The listing builds one solid part. Answer for the finished solid, in the listing's coordinates (mm). A direction names the side the tool comes from. Coordinates: 2 decimals unless noted, no trailing zeros. Write each loop counter-clockwise with the first axis right and the second up, starting at its lowest first coordinate (ties: lowest second). Pieces come first, ordered by that corner, then holes.
(1) Which of the six approach directions +Z, -Z, +X, -X, +Y, -Y give full straight-line access (tool end or side, diameter ignored) to faces 1 (the flat face through (36.512, 6, 129)), 2 (the flat face through (38.1, 6, 125))?
(2) The part is cut by section D-D on z = 50.5. Determine the outline of the cut face in (x, y), plus the area to 3 significant figures.
(3) The part is cut by section B-B on x = 20. Determine the outline of the cut face in (y, z).
(4) The part is cut by section A-A on x = 7. Determine the outline of the cut face in (y, z), plus the area to 3 significant figures.
(5) Straight lines are drawn through the part: line 1 (X direction, y = 8.25, z = 152); line 2 (Y direction, x = 16.5, z = 80.5). For each, find the intervals that lie inside material, in ascending order.
(6) The part is cut by section C-C on y = 5.5. Determine the outline of the cut face in (x, z).
(7) For a pull along X with two mould halves and no side action, classify faces 3 (the flat face through (0, 6, 125)), 4 (the flat face through (18, 1, 0)), 5 (the flat face through (19, 11.112, 129)) as +X half, -X half, draft (parallel to the pull), parting line (faces both ways), or undercut.
from build123d import *

# Parameters (mm, degrees)
SKETCH1_W           = 38.1
SKETCH1_H           = 12.7
BOSS_EXTRUDE1_DEPTH = 254
SKETCH2_W           = 34.925
SKETCH2_H           = 9.525
CUT_EXTRUDE1_DEPTH  = 258.155400488
CUT_EXTRUDE2_DEPTH  = 258.155400488


with BuildPart() as part:
    # Sketch1 → Boss-Extrude1 (new body)
    with BuildSketch(Plane.XY):
        with Locations((19.05, 6.35)):
            Rectangle(SKETCH1_W, SKETCH1_H)
    extrude(amount=BOSS_EXTRUDE1_DEPTH)

    # Sketch2 → Cut-Extrude1 (cut, through all)
    with BuildSketch(Plane.XY.offset(254)):
        with Locations((19.05, 6.35)):
            Rectangle(SKETCH2_W, SKETCH2_H)
    extrude(amount=-CUT_EXTRUDE1_DEPTH, mode=Mode.SUBTRACT)

    # Sketch3 → Cut-Extrude2 (cut, through all)
    with BuildSketch(Plane.XZ):
        Polygon((26.382348419, 241.3), (22.716174209, 247.65), (15.383825791, 247.65), (11.717651581, 241.3), (15.383825791, 234.95), (22.716174209, 234.95), align=None)
    extrude(amount=-CUT_EXTRUDE2_DEPTH, mode=Mode.SUBTRACT)


solid = part.part
Model answer:
1. face 1: +Z, -Z
1. face 2: +Z, -Z, +X, +Y, -Y
2. outline: (0, 0) - (38.1, 0) - (38.1, 12.7) - (0, 12.7) - close; hole (1.59, 1.59) - (36.51, 1.59) - (36.51, 11.11) - (1.59, 11.11) - close
2. area: 151 mm2
3. outline: (0, 0) - (1.59, 0) - (1.59, 234.95) - (0, 234.95) - close; (0, 247.65) - (1.59, 247.65) - (1.59, 254) - (0, 254) - close; (11.11, 0) - (12.7, 0) - (12.7, 234.95) - (11.11, 234.95) - close; (11.11, 247.65) - (12.7, 247.65) - (12.7, 254) - (11.11, 254) - close
4. outline: (0, 0) - (1.59, 0) - (1.59, 254) - (0, 254) - close; (11.11, 0) - (12.7, 0) - (12.7, 254) - (11.11, 254) - close
4. area: 806 mm2
5. line 1: x = 0 to 1.59, 36.51 to 38.1
5. line 2: y = 0 to 1.59, 11.11 to 12.7
6. outline: (0, 0) - (1.59, 0) - (1.59, 254) - (0, 254) - close; (36.51, 0) - (38.1, 0) - (38.1, 254) - (36.51, 254) - close
7. face 3: -X half
7. face 4: draft
7. face 5: undercut
